```python
from build123d import *

# Parameters (mm, degrees)
SPHERE_ANGLE          = 90
SKETCH_R              = 15
PAD_DEPTH             = 25
SKETCH001_R           = 15
PAD001_DEPTH          = 25
SKETCH002_R           = 18
PAD002_DEPTH          = 3
SKETCH003_R           = 18
PAD003_DEPTH          = 3
PAD004_DEPTH          = 1.5
POLARPATTERN_COUNT    = 6
PAD005_DEPTH          = 1.5
POLARPATTERN001_COUNT = 6
SKETCH010_W           = 18
SKETCH010_H           = 10
POCKET_DEPTH          = 18
SKETCH011_R           = 10
POCKET001_DEPTH       = 3
SKETCH012_R           = 10
POCKET002_DEPTH       = 3


with BuildPart() as part:
    # Sphere → Sphere (revolve)
    with BuildSketch(Plane.XZ):
        with BuildLine():
            ThreePointArc((0, -15), (15, 0), (0, 15))
            Line((0, 15), (0, -15))
        make_face()
    revolve(axis=Axis((0, 0, 0), (0, 0, 1)), revolution_arc=SPHERE_ANGLE)

    # Sketch (on Face2 of Sphere) → Pad (new body)
    with BuildSketch(Plane.XZ):
        Circle(SKETCH_R)
    extrude(amount=PAD_DEPTH)

    # Sketch001 (on Face2 of Pad) → Pad001 (join)
    with BuildSketch(Plane(origin=(0, 0, 0), x_dir=(0, -1, 0), z_dir=(-1, 0, 0))):
        Circle(SKETCH001_R)
    extrude(amount=PAD001_DEPTH)

    # Sketch002 (on Face4 of Pad001) → Pad002 (join)
    with BuildSketch(Plane(origin=(-25, 0, 0), x_dir=(0, -1, 0), z_dir=(-1, 0, 0))):
        Circle(SKETCH002_R)
    extrude(amount=PAD002_DEPTH)

    # Sketch003 (on Face7 of Pad002) → Pad003 (join)
    with BuildSketch(Plane.XZ.offset(25)):
        Circle(SKETCH003_R)
    extrude(amount=PAD003_DEPTH)

    # Sketch004 (on Face2 of Pad003) → Pad004 (join)
    with BuildSketch(Plane(origin=(0, -25, 0), x_dir=(-1, 0, 0), z_dir=(0, 1, 0))):
        Polygon((-1.11579, 17.121659), (-0.012041, 17.758909), (1.091708, 17.121659), (1.091708, 15.84716), (-0.012041, 15.209911), (-1.11579, 15.84716), align=None)
    pad004 = extrude(amount=PAD004_DEPTH)

    # PolarPattern: Pad004 ×6 about axis
    polarpattern_axis = Axis((0, -25, 0), (0, 1, 0))
    for i in range(1, POLARPATTERN_COUNT):
        add(pad004.rotate(polarpattern_axis, i * 360 / POLARPATTERN_COUNT))

    # Sketch009 (on Face49 of PolarPattern) → Pad005 (join)
    with BuildSketch(Plane.YZ.offset(-25)):
        Polygon((-1.11579, 17.121659), (-0.012041, 17.758909), (1.091708, 17.121659), (1.091708, 15.84716), (-0.012041, 15.209911), (-1.11579, 15.84716), align=None)
    pad005 = extrude(amount=PAD005_DEPTH)

    # PolarPattern001: Pad005 ×6 about axis
    polarpattern001_axis = Axis((-25, 0, 0), (1, 0, 0))
    for i in range(1, POLARPATTERN001_COUNT):
        add(pad005.rotate(polarpattern001_axis, i * 360 / POLARPATTERN001_COUNT))

    # Sketch010 (on Face3 of PolarPattern001) → Pocket (cut)
    with BuildSketch(Plane.XZ.offset(28)):
        with Locations((-19, 0)):
            Rectangle(SKETCH010_W, SKETCH010_H)
    extrude(amount=-POCKET_DEPTH, mode=Mode.SUBTRACT)

    # Sketch011 (on Face4 of Pocket) → Pocket001 (cut)
    with BuildSketch(Plane.XZ.offset(28)):
        Circle(SKETCH011_R)
    extrude(amount=-POCKET001_DEPTH, mode=Mode.SUBTRACT)

    # Sketch012 (on Face50 of Pocket001) → Pocket002 (cut)
    with BuildSketch(Plane(origin=(-28, 0, 0), x_dir=(0, -1, 0), z_dir=(-1, 0, 0))):
        Circle(SKETCH012_R)
    extrude(amount=-POCKET002_DEPTH, mode=Mode.SUBTRACT)


solid = part.part
```
The model under review builds one solid part; all positions refer to its coordinate system, in mm. A direction names the side the tool comes from. Round coordinates to 2 decimals unless told otherwise and drop trailing zeros. Write each loop counter-clockwise with the first axis right and the second up, starting at its lowest first coordinate (ties: lowest second). Pieces come first, ordered by that corner, then holes. Notation, with made-up numbers: M 20.25,21 L 66.25,21 A17 ccw 66.25,40 Z; hole C -26,-16 d11. An arc over 180 degrees is marked long. Use CSV: the item, a comma, the result in double quotes. Start each with the question number.
(1) For line 1 along Z through (x, y) = (-26.85, 0); line 2 along Z through (x, y) = (-20.5, -13); line 3 along Y through (x, z) = (10.5, -14.5), list the stretches that pass through material, from the lowest coordinate up.
(2) Clearance check with flat-ended pins moving along their axes: P1, Ø5, axis at x = 7, z = -6, coming from the +Y side; P2, Ø12, axis at x = 13, z = 14.5, coming from the +Y side; P3, Ø5, axis at x = -8, y = 6, coming from the +Z side. State where each tip first meets the part, or that it passes through.
(3) We need section A-A, the plane x = 7.5. State the section outline as (y, z) points, then the cut area to 3 significant figures.
(4) We need section C-C, the plane x = -21. State the section outline as (y, z) points, then the cut area to 3 significant figures.
(5) The part is to be moulded in two halves that separate along Y. For faces 1 (the face through (15.386, -24, 8)), 2 (the face through (-24, -1.116, 16)), 3 (the face through (-24, 13.178, -8)), say which applies: +Y half, -Y half, draft (parallel to the pull), parting line (faces both ways), or undercut.
(6) Tool access review of faces 4 (the face through (13.166, -24, -8)), 5 (the face through (0, -23.5, 17)), 6 (the face through (-24, -13.166, -8)), 7 (the face through (14, -23.5, -8)), 8 (the face through (-26.52, 2.17, -9.76)): name each direction out of +Z, -Z, +X, -X, +Y, -Y from which nothing blocks a thin tool from reaching the whole face with its end or side.
(7) We need section B-B, the plane z = -12. State the section outline as (x, y) points.
Findings:
1,line 1,"-18 to -10, 10 to 18"
1,line 2,"-7.48 to -5, 5 to 7.48"
1,line 3,"-28 to -25"
2,P1,"y = 13.41"
2,P2,"y = 6.59"
2,P3,"z = 14.59"
3,outline,"M -28,-16.36 L -25,-16.36 L -25,-12.99 L 0,-12.99 A12.99 ccw 0,12.99 L -25,12.99 L -25,16.36 L -28,16.36 L -28,6.61 L -25,6.61 L -25,-6.61 L -28,-6.61 Z"
3,area,"973 mm^2"
4,outline,"M -14.14,-5 A15 ccw long -14.14,5 L -10,5 L -10,-5 Z"
4,area,"660 mm^2"
5,face 1,"draft"
5,face 2,"-Y half"
5,face 3,"undercut"
6,face 4,"-Z, +Y"
6,face 5,"+Z, +X, -X, +Y"
6,face 6,"-Z"
6,face 7,"-Z, +X, +Y"
6,face 8,"-X"
7,outline,"M -28,-13.42 L -25,-13.42 L -25,-9 L -9,-9 L -9,-25 L -13.42,-25 L -13.42,-28 L 13.42,-28 L 13.42,-25 L 9,-25 L 9,0 A9 ccw 0,9 L -25,9 L -25,13.42 L -28,13.42 Z"
